CAD build for the part. Positions are in the model's coordinates, mm. Coordinates: 2 decimals unless noted, no trailing zeros. Write each loop counter-clockwise with the first axis right and the second up, starting at its lowest first coordinate (ties: lowest second). Pieces come first, ordered by that corner, then holes. Notation, with made-up numbers: (89, -1.75) -> (104, -1.75) arc R16 cw to (104, 6.25) -> close; hole circle Ø11 at (75, -9). An arc over 180 degrees is marked (long way). Answer as CSV lines item,"result".
```python
from build123d import *

# Parameters (mm, degrees)
SKETCH1_W                   = 76.2
SKETCH1_H                   = 25.4
EXTRUDE1_DEPTH              = 6.35
F_3_8_CLEARANCE_HOLE1_D     = 10.0838
F_3_8_CLEARANCE_HOLE1_DEPTH = 16.002
F_3_8_CLEARANCE_HOLE1_TIP   = 3.029479155


with BuildPart() as part:
    # Sketch1 → Extrude1 (new body)
    with BuildSketch(Plane.XY):
        Rectangle(SKETCH1_W, SKETCH1_H)
    extrude(amount=EXTRUDE1_DEPTH)

    # 3/8 Clearance Hole1
    with Locations(Plane(origin=(25.4, 0, 6.35), x_dir=(1, 0, 0), z_dir=(0, 0, 1))):
        with Locations((0, 0)):
            Hole(F_3_8_CLEARANCE_HOLE1_D / 2, depth=F_3_8_CLEARANCE_HOLE1_DEPTH)
            with Locations((0, 0, -(F_3_8_CLEARANCE_HOLE1_DEPTH + F_3_8_CLEARANCE_HOLE1_TIP / 2))):  # 118° drill point
                Cone(0, F_3_8_CLEARANCE_HOLE1_D / 2, F_3_8_CLEARANCE_HOLE1_TIP, mode=Mode.SUBTRACT)


solid = part.part
```
Item 1: Saw through at B-B on y = 0. Give the cut face in (x, z), and give its area (3 significant figures).
Answer below:
outline,"(-38.1, 0) -> (20.36, 0) -> (20.36, 6.35) -> (-38.1, 6.35) -> close; (30.44, 0) -> (38.1, 0) -> (38.1, 6.35) -> (30.44, 6.35) -> close"
area,"420 mm2"
Item 2: Flat gauge pins, fed straight in: pin 1 (5 mm diameter, centred on x = 20.5, y = 9.5, fed in from -Z); pin 2 (9 mm diameter, centred on x = 25.4, y = 0, fed in from -Z). Where does each tip first touch, or does it go through?
Answer below:
pin 1,"stops at z = 0"
pin 2,"passes through"
Item 3: Saw through at A-A on x = 25.4. Give the cut face in (y, z).
Answer below:
outline,"(-12.7, 0) -> (-5.04, 0) -> (-5.04, 6.35) -> (-12.7, 6.35) -> close; (5.04, 0) -> (12.7, 0) -> (12.7, 6.35) -> (5.04, 6.35) -> close"
Item 4: Saw through at C-C on z = 1.5. Give the cut face in (x, y), and give its area (3 significant figures).
Answer below:
outline,"(-38.1, -12.7) -> (38.1, -12.7) -> (38.1, 12.7) -> (-38.1, 12.7) -> close; hole circle Ø10.08 at (25.4, 0)"
area,"1,860 mm2"
Item 5: Wall check: line 1 (Y direction, x = 25.4, z = 3.25); line 2 (X direction, y = 2, z = 5.25); line 3 (Y direction, x = 24, z = 1). Give the ranges that are in metal, low to high. Write a range as from..to.
Answer below:
line 1,"y = -12.7..-5.04, 5.04..12.7"
line 2,"x = -38.1..20.77, 30.03..38.1"
line 3,"y = -12.7..-4.84, 4.84..12.7"
Item 6: Two-plate mould, pull along Y, no slides. Class faces 1 (the cylindrical face through (20.74, -1.93, 3.13)), 2 (the flat face through (-1, 12.7, 3)), 3 (the flat face through (-1, -12.7, 3)): pulls with the +Y half, pulls with the -Y half, needs draft (parallel to the pull), parting line crosses it, or undercut.
Answer below:
face 1,"undercut"
face 2,"pulls with the +Y half"
face 3,"pulls with the -Y half"
